Source: three-view drawing plus pictorial views. Frame: mm from the lowest corner of the part. Coordinates: 2 decimals unless noted, no trailing zeros. Loops run counter-clockwise (first coordinate to the right, second up) from the corner with the lowest first, then second, coordinate; pieces in that order, holes last.
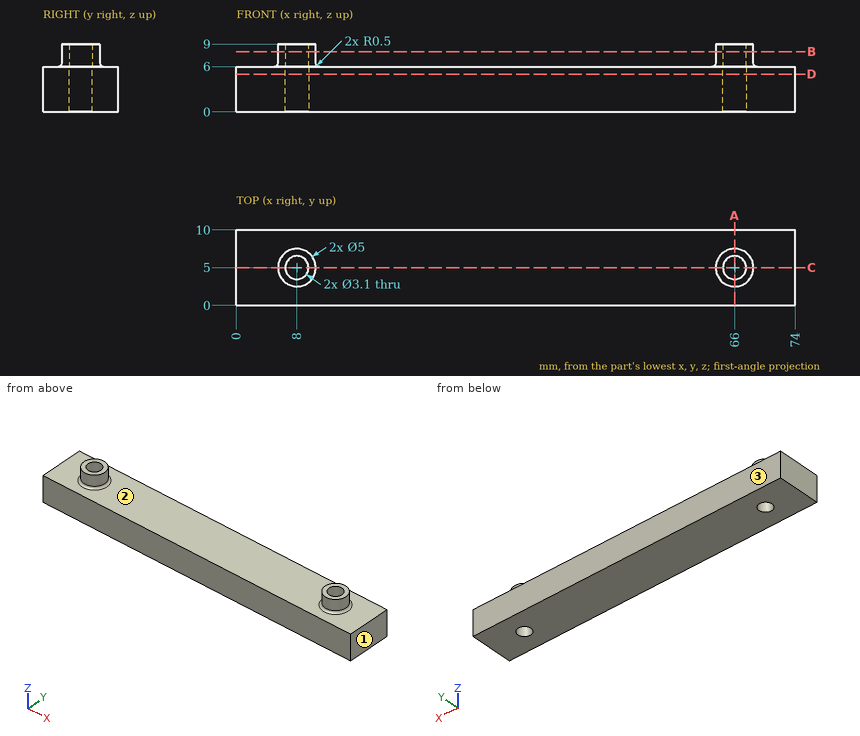
Q1. Material intervals for line 1 along Y through (x, z) = (66, 7.15); line 2 along X through (y, z) = (5.75, 6.5); line 3 along X through (y, z) = (5.5, 1.5), sorted ascending.
Q2. Draft query along X for the marked faces 1, 2 and 3. Return one class per face: released by +X, released by -X, zero draft, split by the parting line, or undercut.
Q3. Section query D-D on z = 5. Return the cut outline in (x, y).
Q4. Section query A-A on x = 66. Return the cut outline in (y, z).
Q5. Section query B-B on z = 8. Return the cut outline in (x, y).
Q6. Section query C-C on y = 5. Return the cut outline in (x, z), then the cut area to 3 significant figures.
Q7. First-contact query: pin 1 Ø2 at (x, z) = (39, 5) entering from -Y; pin 2 Ø3 at (x, y) = (25, 5.5) entering from +Z. Flat tips, straight axial feed; report the tip coordinate or a pass-through.
Resolved:
1. line 1: y = 2.5 to 3.45, 6.55 to 7.5
1. line 2: x = 5.62 to 6.64, 9.36 to 10.38, 63.62 to 64.64, 67.36 to 68.38
1. line 3: x = 0 to 6.53, 9.47 to 64.53, 67.47 to 74
2. face 1: released by +X
2. face 2: undercut
2. face 3: zero draft
3. outline: (0, 0) - (74, 0) - (74, 10) - (0, 10) - close; hole circle Ø3.1 at (8, 5); hole circle Ø3.1 at (66, 5)
4. outline: (0, 0) - (3.45, 0) - (3.45, 9) - (2.5, 9) - (2.5, 6.5) arc R0.5 cw to (2, 6) - (0, 6) - close; (6.55, 0) - (10, 0) - (10, 6) - (8, 6) arc R0.5 cw to (7.5, 6.5) - (7.5, 9) - (6.55, 9) - close
5. outline: circle Ø5 at (8, 5); circle Ø5 at (66, 5); hole circle Ø3.1 at (8, 5); hole circle Ø3.1 at (66, 5)
6. outline: (0, 0) - (6.45, 0) - (6.45, 9) - (5.5, 9) - (5.5, 6.5) arc R0.5 cw to (5, 6) - (0, 6) - close; (9.55, 0) - (64.45, 0) - (64.45, 9) - (63.5, 9) - (63.5, 6.5) arc R0.5 cw to (63, 6) - (11, 6) arc R0.5 cw to (10.5, 6.5) - (10.5, 9) - (9.55, 9) - close; (67.55, 0) - (74, 0) - (74, 6) - (69, 6) arc R0.5 cw to (68.5, 6.5) - (68.5, 9) - (67.55, 9) - close
6. area: 418 mm2
7. pin 1: stops at y = 0
7. pin 2: stops at z = 6
